Here's the drawing with two shaded views (mm, measured from the low corner). I have some questions. Round coordinates to 2 decimals unless told otherwise and drop trailing zeros. Order: outer loops, then holes, each group sorted by start corner. A loop starts at its lowest first (then second) coordinate and runs counter-clockwise, first axis right, second up.
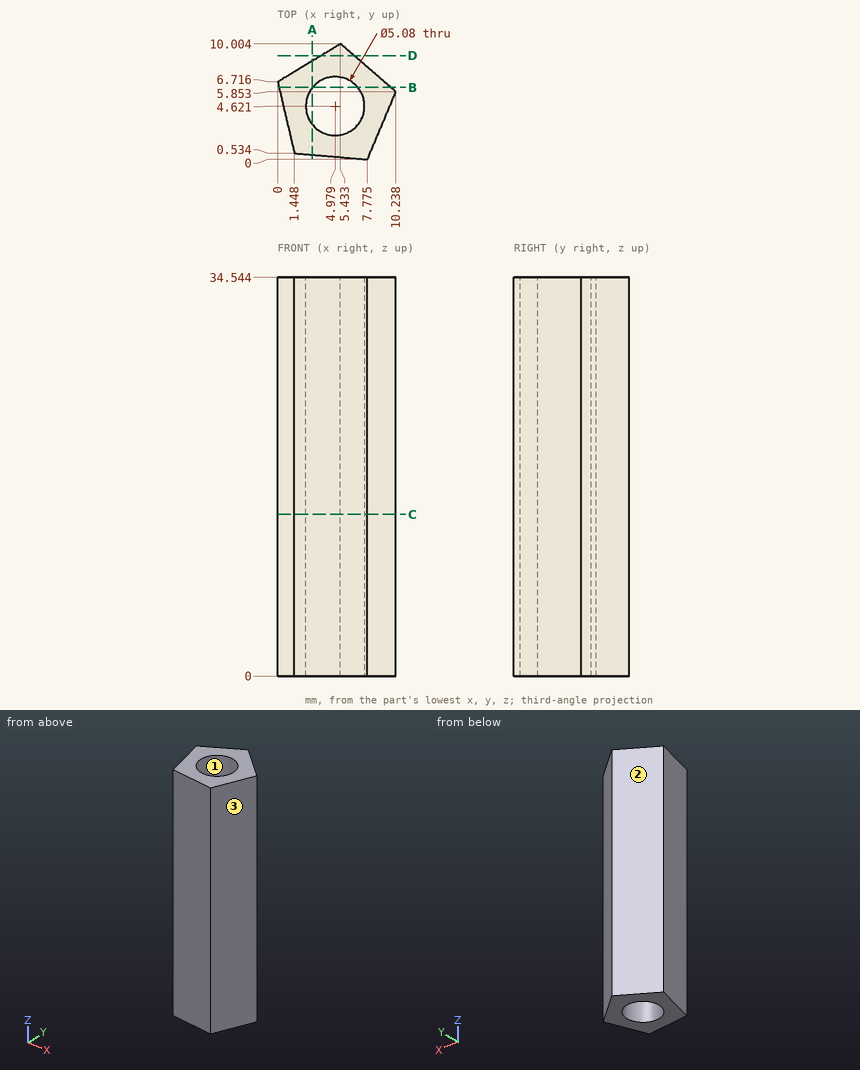
1. If we mould it in two halves opening along Y, with no side actions, what happens to the marked faces 1, 2 and 3? For each: released by +Y, released by -Y, zero draft, split by the parting line, or undercut.
Evaluation:
face 1: undercut
face 2: released by +Y
face 3: released by -Y
2. If we section it at D-D, the plane y = 9: Write out the boundary of the cut face in (x, z) (1 decimal).
Evaluation:
outline: (3.8, 0) - (6.6, 0) - (6.6, 34.5) - (3.8, 34.5) - close
3. I need wall thicknesses on probe 1 along Y at (x, z) = (7.25, 12.5) (1 decimal); probe 2 along X at (y, z) = (4, 18) (1 decimal); probe 3 along Y at (x, z) = (3.5, 32.5) (1 decimal). Which ranges of each line are inside material? Lowest first, please.
Evaluation:
probe 1: y = 0 to 3.5, 5.8 to 8.4
probe 2: x = 0.6 to 2.5, 7.4 to 9.5
probe 3: y = 0.4 to 2.6, 6.7 to 8.8
4. If we section it at B-B, the plane y = 6.25: Write out the boundary of the cut face in (x, z).
Evaluation:
outline: (0.11, 0) - (3.03, 0) - (3.03, 34.54) - (0.11, 34.54) - close; (6.93, 0) - (9.78, 0) - (9.78, 34.54) - (6.93, 34.54) - close
5. If we section it at C-C, the plane z = 14: Write out the boundary of the cut face in (x, y) (1 decimal).
Evaluation:
outline: (0, 6.7) - (1.4, 0.5) - (7.8, 0) - (10.2, 5.9) - (5.4, 10) - close; hole circle Ø5.1 at (5, 4.6)
6. I'm going to push flat-ended pins straight in: P1, Ø3, axis at y = 7, z = 8, coming from the +X side; P2, Ø3, axis at x = 4.98, y = 4.62, coming from the -Z side; P3, Ø1.5, axis at y = 2, z = 29.5, coming from the -X side; P4, Ø4, axis at y = 2.5, z = 24.5, coming from the -X side. Where does each tip first touch, or does it pass through?
Evaluation:
P1: stops at x = 10.24
P2: passes through
P3: stops at x = 0.93
P4: stops at x = 0.52
7. If we section it at A-A, the plane x = 3: Write out the boundary of the cut face in (y, z), and give its area (3 significant figures).
Evaluation:
outline: (0.4, 0) - (3.03, 0) - (3.03, 34.54) - (0.4, 34.54) - close; (6.21, 0) - (8.53, 0) - (8.53, 34.54) - (6.21, 34.54) - close
area: 171 mm2
